Design review of the part shown in the three views and the two pictorial views. Dimensions are in mm from the part's minimum x, y and z. Give positions to 0.01 mm unless a question says otherwise; leave off trailing zeros. Write each loop counter-clockwise with the first axis right and the second up, starting at its lowest first coordinate (ties: lowest second). Pieces come first, ordered by that corner, then holes. Notation, with made-up numbers: (-5, 83.5) -> (6, 83.5) arc R20 ccw to (6, 121.5) -> close; hole circle Ø5 at (41.5, -23). An arc over 180 degrees is marked (long way). Use CSV: the item, a comma, the result in double quotes.
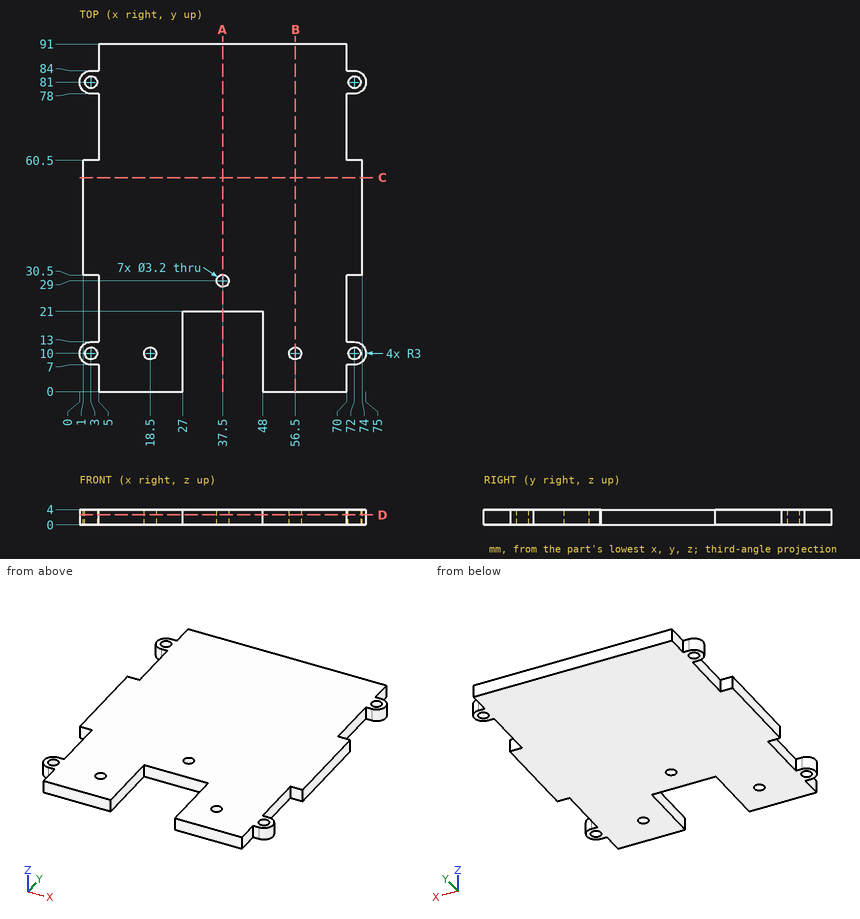
Q1. Consider section D-D (z = 2.6). State how many separate pieces and enclosed holes the cut face has, then the cut area to 3 significant figures.
Derived:
separate pieces,"1"
enclosed holes,"7"
area,"5,760 mm2"
Q2. To check wall thickness, follow probe 1 along Y at (x, z) = (72, 1.65); probe 2 along X at (y, z) = (81, 1.9); probe 3 along Y at (x, z) = (56.5, 1.55). State the ranges of each line that lie inside material, in increasing order.
Derived:
probe 1,"y = 7 to 8.4, 11.6 to 13, 30.5 to 60.5, 78 to 79.4, 82.6 to 84"
probe 2,"x = 0 to 1.4, 4.6 to 70.4, 73.6 to 75"
probe 3,"y = 0 to 8.4, 11.6 to 91"
Q3. Insertion check: pin 1 (1.2 mm diameter, centred on x = 3.5, z = 2, fed in from +Y); pin 2 (1.2 mm diameter, centred on y = 20.5, z = 2, fed in from -X); pin 3 (1.2 mm diameter, centred on y = 47.5, z = 2, fed in from +X). Each pin has a flat end and moves straight along its axis. Give the tip position at first contact, or say it passes through.
Derived:
pin 1,"stops at y = 84"
pin 2,"stops at x = 5"
pin 3,"stops at x = 74"
Q4. Consider section A-A (x = 37.5). Write out the cut boundary in (y, z), then the cut area to 3 significant figures.
Derived:
outline,"(21, 0) -> (27.4, 0) -> (27.4, 4) -> (21, 4) -> close; (30.6, 0) -> (91, 0) -> (91, 4) -> (30.6, 4) -> close"
area,"267 mm2"
Q5. Consider section B-B (x = 56.5). Write out the cut boundary in (y, z), then the cut area to 3 significant figures.
Derived:
outline,"(0, 0) -> (8.4, 0) -> (8.4, 4) -> (0, 4) -> close; (11.6, 0) -> (91, 0) -> (91, 4) -> (11.6, 4) -> close"
area,"351 mm2"
Q6. Consider section C-C (y = 56). Write out the cut boundary in (x, z), then the cut area to 3 significant figures.
Derived:
outline,"(1, 0) -> (74, 0) -> (74, 4) -> (1, 4) -> close"
area,"292 mm2"
